Design review of the part built by this model. Coordinates are the model's own, in mm. Round coordinates to 2 decimals unless told otherwise and drop trailing zeros. Write each loop counter-clockwise with the first axis right and the second up, starting at its lowest first coordinate (ties: lowest second). Pieces come first, ordered by that corner, then holes. Notation, with made-up numbers: (9, -15) -> (31, -15) arc R22 cw to (31, 12) -> close; hole circle Ø1 at (-4.5, -5.75). An arc over 180 degrees is marked (long way). Write item = value, one per line. Start each with the question number.
Item 1: To check wall thickness, follow L1, parallel to X at y = 22.5, z = 21.5; L2, parallel to X at y = -21, z = 9; L3, parallel to X at y = -20.5, z = 8. State the ranges of each line that lie inside material, in increasing order.
Item 2: Add section B-B, the plane x = 154.5. State the section outline as (y, z) points.
Item 3: Add section A-A, the plane z = 16.25. State the section outline as (x, y) points.
Item 4: For pin 1 Ø8 at (y, z) = (15, 4.5) entering from +X; pin 2 Ø3 at (x, z) = (156, 9) entering from +Y, all flat-tipped, find the tip position at first contact; note any pin that passes through.
from build123d import *

# Parameters (mm, degrees)
EXTRUDE_1_DEPTH        = 25
SKETCH_2_W             = 115
SKETCH_2_H             = 6
CUT_EXTRUDE_1_DEPTH    = 7.5
MIRROR_START           = 6
MIRROR_1_DEPTH         = 6
PATTERN_LINEAR_1_COUNT = 2
PATTERN_LINEAR_1_PITCH = 1750
CUT_EXTRUDE_2_REACH    = 2492.351


# Read off the part's stored shape, not the designer's step: 镜向1
with BuildPart() as part:
    # 草图1 → 凸台-拉伸1 (new body)
    with BuildSketch(Plane.XY):
        Polygon((0, 24), (0, -24), (2295, -24), (2295, -9.5), (2490, -9.5), (2490, 9.5), (2295, 9.5), (2295, 24), align=None)
    extrude(amount=EXTRUDE_1_DEPTH)

    # 草图2 → 切除-拉伸1 (cut)
    with BuildSketch(Plane.XZ.offset(24)):
        with Locations((1900, 9)):
            Rectangle(SKETCH_2_W, SKETCH_2_H)
    cut_extrude_1 = extrude(amount=-CUT_EXTRUDE_1_DEPTH, mode=Mode.SUBTRACT)

    # 镜向1 outline → 镜向1 (cut)
    with BuildSketch(Plane.XY.offset(MIRROR_START)):
        Polygon((1842.5, 16.5), (1957.5, 16.5), (1965, 24), (1835, 24), align=None)
        Polygon((1835, -24), (1842.5, -24), (1842.5, -16.5), align=None)
        Polygon((1965, -24), (1957.5, -16.5), (1957.5, -24), align=None)
    mirror_1 = extrude(amount=MIRROR_1_DEPTH, mode=Mode.SUBTRACT)

    # 阵列(线性)1: 切除-拉伸1, 镜向1 ×2
    with Locations(*[(-i * PATTERN_LINEAR_1_PITCH, 0, 0) for i in range(1, PATTERN_LINEAR_1_COUNT)]):
        add(cut_extrude_1, mode=Mode.SUBTRACT)
        add(mirror_1, mode=Mode.SUBTRACT)

    # 草图3 → 切除-拉伸2 (cut, up to next)
    with BuildSketch(Plane.XZ.offset(9.5), mode=Mode.PRIVATE) as cut_extrude_2_sk1:
        Polygon((2400, 25), (2490, 10), (2490, 25), align=None)
    cut_extrude_2_tool1 = extrude(cut_extrude_2_sk1.sketch, amount=-CUT_EXTRUDE_2_REACH, mode=Mode.PRIVATE) & part.part
    add(cut_extrude_2_tool1.solids().sort_by_distance((2460, -9.5, 20))[0], mode=Mode.SUBTRACT)


solid = part.part
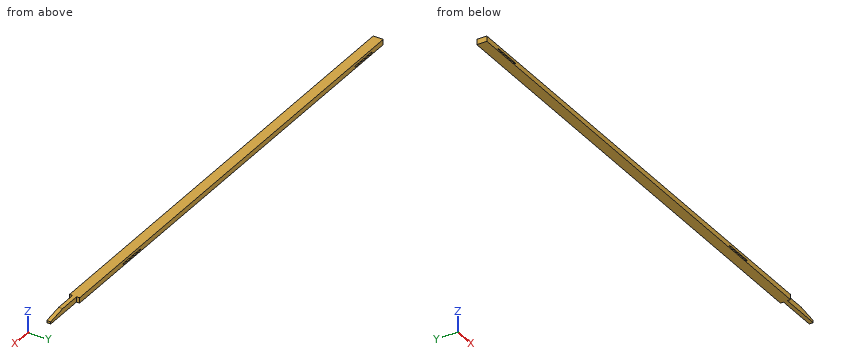
Result set:
q1.L1 = 0 to 2295
q1.L2 = 0 to 88, 212 to 1838, 1962 to 2295
q1.L3 = 0 to 88.5, 211.5 to 1838.5, 1961.5 to 2295
q2.outline = (-24, 0) -> (24, 0) -> (24, 6) -> (16.5, 6) -> (16.5, 12) -> (24, 12) -> (24, 25) -> (-24, 25) -> (-24, 12) -> (-16.5, 12) -> (-16.5, 6) -> (-24, 6) -> close
q3.outline = (0, -24) -> (2295, -24) -> (2295, -9.5) -> (2452.5, -9.5) -> (2452.5, 9.5) -> (2295, 9.5) -> (2295, 24) -> (0, 24) -> close
q4.pin_1 = 2295
q4.pin_2 = 16.5
